For this review, take the finished solid that the model builds, in its own axes (mm). A direction names the side the tool comes from. Coordinates: 2 decimals unless noted, no trailing zeros. Order: outer loops, then holes, each group sorted by start corner. A loop starts at its lowest first (then second) coordinate and runs counter-clockwise, first axis right, second up. Notation, with made-up numbers: (82, 71.5) - (112, 71.5) arc R26 cw to (112, 100.5) - close; hole circle Ø2 at (45.25, 86.5). An arc over 180 degrees is marked (long way). One line per item, written item: value. Start each with the question number.
(1) For faces 1 (the flat face through (37.27, 27.014, -76.545)), 2 (the flat face through (135, 14, -62)), 3 (the flat face through (37.581, 27.014, -8.694)), list the 3-axis set-ups (+Z, -Z, +X, -X, +Y, -Y) from which the entire face can be reached by the end or side of a thin tool; tool diameter is ignored.
(2) Consider section B-B on z = -72. Write out the cut boundary in (x, y), then the cut area to 3 significant figures.
(3) Mouldability with a two-part tool opening along X and no side actions: class faces 4 (the flat face through (72, 14, -85)), 5 (the flat face through (147, 14, -31)), 6 (the flat face through (76, 26, -77)) as released by +X, released by -X, zero draft, split by the parting line, or undercut.
(4) To check wall thickness, follow line 1 along X through (y, z) = (22, -56.5); line 2 along Y through (x, z) = (36.5, -4.5); line 3 along X through (y, z) = (14, -63). State the ranges of each line that lie inside material, in increasing order.
(5) Consider section A-A on x = 77.5. Write out the cut boundary in (y, z), then the cut area to 3 significant figures.
(6) Clearance check with flat-ended pins moving along their axes: pin 1 (1 mm diameter, centred on y = 26.5, z = -79.5, fed in from -X); pin 2 (1.6 mm diameter, centred on y = 27, z = -80.5, fed in from +X); pin 3 (2 mm diameter, centred on y = 23, z = -35, fed in from +X). State where each tip first meets the part, or that it passes through.
```python
from build123d import *

# Parameters (mm, degrees)
SKETCH2_W           = 145
SKETCH2_H           = 85
BOSS_EXTRUDE1_DEPTH = 28
FILLET1_R           = 2.5
SKETCH3_R           = 2.115255866
CUT_EXTRUDE1_DEPTH  = 10
SKETCH4_W           = 20.962420857
SKETCH4_H           = 9.466899742
BOSS_EXTRUDE2_DEPTH = 2
CUT_EXTRUDE2_DEPTH  = 2


with BuildPart() as part:
    # Sketch2 → Boss-Extrude1 (new body)
    with BuildSketch(Plane(origin=(0, 0, 0), x_dir=(1, 0, 0), z_dir=(0, 1, 0))):
        with Locations((72.5, 42.5)):
            Rectangle(SKETCH2_W, SKETCH2_H)
    extrude(amount=BOSS_EXTRUDE1_DEPTH)

    # Fillet1
    fillet1_edges = [part.edges().sort_by_distance(p)[0] for p in [
        (145, 28, -42.5),
        (72.5, 28, -85),
        (0, 28, -42.5),
        (72.5, 0, -85),
        (145, 0, -42.5),
        (72.5, 0, 0),
        (0, 0, -42.5),
        (0, 14, -85),
        (145, 14, -85),
        (145, 14, 0),
        (0, 14, 0),
        (72.5, 28, 0),
    ]]
    fillet(fillet1_edges, radius=FILLET1_R)

    # Sketch3 → Cut-Extrude1 (cut)
    with BuildSketch(Plane(origin=(145, 0, 0), x_dir=(0, 0, -1), z_dir=(1, 0, 0))):
        with Locations((62.355900108, 14.02082484)):
            Circle(SKETCH3_R)
    extrude(amount=-CUT_EXTRUDE1_DEPTH, mode=Mode.SUBTRACT)

    # Sketch4 → Boss-Extrude2 (add)
    with BuildSketch(Plane(origin=(145, 0, 0), x_dir=(0, 0, -1), z_dir=(1, 0, 0))):
        with Locations((31.281109073, 14.236048875)):
            Rectangle(SKETCH4_W, SKETCH4_H)
    extrude(amount=BOSS_EXTRUDE2_DEPTH)

    # Sketch5 → Cut-Extrude2 (cut)
    with BuildSketch(Plane(origin=(0, 28, 0), x_dir=(1, 0, 0), z_dir=(0, 1, 0))):
        with BuildLine():
            Line((26.254495466, 85), (48.530276138, 67.90157817))
            Line((48.530276138, 67.90157817), (102.643480063, 67.90157817))
            Line((102.643480063, 67.90157817), (126.477007635, 85))
            Line((126.477007635, 85), (101.67856471, 85))
            Line((101.67856471, 85), (101.67856471, 77.955286257))
            ThreePointArc((101.67856471, 77.955286257), (100.949025715, 77.225747261), (100.21948672, 77.955286257))
            Line((100.21948672, 77.955286257), (100.21948672, 85))
            Line((100.21948672, 85), (91.67856471, 85))
            Line((91.67856471, 85), (91.67856471, 77.955286257))
            ThreePointArc((91.67856471, 77.955286257), (90.949025715, 77.225747261), (90.21948672, 77.955286257))
            Line((90.21948672, 77.955286257), (90.21948672, 85))
            Line((90.21948672, 85), (81.67856471, 85))
            Line((81.67856471, 85), (81.67856471, 77.955286257))
            ThreePointArc((81.67856471, 77.955286257), (80.949025715, 77.225747261), (80.21948672, 77.955286257))
            Line((80.21948672, 77.955286257), (80.21948672, 85))
            Line((80.21948672, 85), (71.67856471, 85))
            Line((71.67856471, 85), (71.67856471, 77.955286257))
            ThreePointArc((71.67856471, 77.955286257), (70.949025715, 77.225747261), (70.21948672, 77.955286257))
            Line((70.21948672, 77.955286257), (70.21948672, 85))
            Line((70.21948672, 85), (61.67856471, 85))
            Line((61.67856471, 85), (61.67856471, 77.955286257))
            ThreePointArc((61.67856471, 77.955286257), (60.949025715, 77.225747261), (60.21948672, 77.955286257))
            Line((60.21948672, 77.955286257), (60.21948672, 85))
            Line((60.21948672, 85), (51.67856471, 85))
            Line((51.67856471, 85), (51.67856471, 77.955286257))
            ThreePointArc((51.67856471, 77.955286257), (50.949025715, 77.225747261), (50.21948672, 77.955286257))
            Line((50.21948672, 77.955286257), (50.21948672, 85))
            Line((50.21948672, 85), (26.254495466, 85))
        make_face()
        with BuildLine():
            Line((101.67856471, 0), (126.477007635, 0))
            Line((126.477007635, 0), (102.643480063, 17.09842183))
            Line((102.643480063, 17.09842183), (48.530276138, 17.09842183))
            Line((48.530276138, 17.09842183), (26.254495466, 0))
            Line((26.254495466, 0), (50.21948672, 0))
            Line((50.21948672, 0), (50.21948672, 7.044713743))
            ThreePointArc((50.21948672, 7.044713743), (50.949025715, 7.774252739), (51.67856471, 7.044713743))
            Line((51.67856471, 7.044713743), (51.67856471, 0))
            Line((51.67856471, 0), (60.21948672, 0))
            Line((60.21948672, 0), (60.21948672, 7.044713743))
            ThreePointArc((60.21948672, 7.044713743), (60.949025715, 7.774252739), (61.67856471, 7.044713743))
            Line((61.67856471, 7.044713743), (61.67856471, 0))
            Line((61.67856471, 0), (70.21948672, 0))
            Line((70.21948672, 0), (70.21948672, 7.044713743))
            ThreePointArc((70.21948672, 7.044713743), (70.949025715, 7.774252739), (71.67856471, 7.044713743))
            Line((71.67856471, 7.044713743), (71.67856471, 0))
            Line((71.67856471, 0), (80.21948672, 0))
            Line((80.21948672, 0), (80.21948672, 7.044713743))
            ThreePointArc((80.21948672, 7.044713743), (80.949025715, 7.774252739), (81.67856471, 7.044713743))
            Line((81.67856471, 7.044713743), (81.67856471, 0))
            Line((81.67856471, 0), (90.21948672, 0))
            Line((90.21948672, 0), (90.21948672, 7.044713743))
            ThreePointArc((90.21948672, 7.044713743), (90.949025715, 7.774252739), (91.67856471, 7.044713743))
            Line((91.67856471, 7.044713743), (91.67856471, 0))
            Line((91.67856471, 0), (100.21948672, 0))
            Line((100.21948672, 0), (100.21948672, 7.044713743))
            ThreePointArc((100.21948672, 7.044713743), (100.949025715, 7.774252739), (101.67856471, 7.044713743))
            Line((101.67856471, 7.044713743), (101.67856471, 0))
        make_face()
    extrude(amount=-CUT_EXTRUDE2_DEPTH, mode=Mode.SUBTRACT)


solid = part.part
```
Geometry check:
1. face 1: -Z, +Y
1. face 2: +X
1. face 3: +Z, +Y
2. outline: (0, 2.5) arc R2.5 ccw to (2.5, 0) - (142.5, 0) arc R2.5 ccw to (145, 2.5) - (145, 25.5) arc R2.5 ccw to (142.5, 28) - (108.36, 28) - (108.36, 26) - (43.19, 26) - (43.19, 28) - (2.5, 28) arc R2.5 ccw to (0, 25.5) - close
2. area: 3,920 mm^2
3. face 4: zero draft
3. face 5: released by +X
3. face 6: undercut
4. line 1: x = 0 to 145
4. line 2: y = 0 to 26
4. line 3: x = 0 to 135
5. outline: (0, -82.5) arc R2.5 ccw to (2.5, -85) - (25.5, -85) arc R2.5 ccw to (26, -84.95) - (26, -67.9) - (28, -67.9) - (28, -17.1) - (26, -17.1) - (26, -0.05) arc R2.5 ccw to (25.5, 0) - (2.5, 0) arc R2.5 ccw to (0, -2.5) - close
5. area: 2,310 mm^2
6. pin 1: stops at x = 0.05
6. pin 2: stops at x = 144.9
6. pin 3: stops at x = 145
